from build123d import *

# Parameters (mm, degrees)
PAD008_DEPTH    = 21
POCKET020_DEPTH = 74.801
POCKET021_DEPTH = 1
CHAMFER008_SIZE = 0.99
POCKET022_DEPTH = 1
CHAMFER009_SIZE = 0.99
POCKET023_DEPTH = 74.801
CHAMFER010_SIZE = 4
FILLET003_R     = 6
FILLET004_R     = 5
SKETCH033_W     = 74.8
SKETCH033_H     = 11
PAD009_DEPTH    = 24
SKETCH034_R     = 3.15
POCKET024_DEPTH = 22.001
SKETCH035_R     = 7.5
POCKET025_DEPTH = 6
CHAMFER011_SIZE = 9
FILLET005_R     = 3
CHAMFER012_SIZE = 0.4


with BuildPart() as part:
    # Sketch028 → Pad008 (new body)
    with BuildSketch(Plane.XY):
        Polygon((-25.65, -11), (-25.65, 0.15), (35.45, 0.15), (35.45, -11), (42.3, -11), (42.3, 11), (-32.5, 11), (-32.5, -11), align=None)
    extrude(amount=PAD008_DEPTH)

    # Sketch029 (on Face7 of Pad008) → Pocket020 (cut, through all)
    with BuildSketch(Plane(origin=(-32.5, 0, 0), x_dir=(0, -1, 0), z_dir=(-1, 0, 0))):
        with BuildLine():
            ThreePointArc((3.35, 6.5), (5, 4.85), (6.65, 6.5))
            Line((6.65, 6.5), (6.65, 11.5))
            ThreePointArc((6.65, 11.5), (5, 13.15), (3.35, 11.5))
            Line((3.35, 6.5), (3.35, 11.5))
        make_face()
    extrude(amount=-POCKET020_DEPTH, mode=Mode.SUBTRACT)

    # Sketch030 (on Face10 of Pocket020) → Pocket021 (cut)
    with BuildSketch(Plane(origin=(-32.5, 0, 0), x_dir=(0, -1, 0), z_dir=(-1, 0, 0))):
        with BuildLine():
            ThreePointArc((8.65, 11.5), (5, 15.15), (1.35, 11.5))
            Line((1.35, 11.5), (1.35, 6.5))
            ThreePointArc((1.35, 6.5), (5, 2.85), (8.65, 6.5))
            Line((8.65, 11.5), (8.65, 6.5))
        make_face()
    extrude(amount=-POCKET021_DEPTH, mode=Mode.SUBTRACT)

    # Chamfer008
    chamfer008_edges = [part.edges().sort_by_distance(p)[0] for p in [
        (-32.5, -1.35, 9),
    ]]
    chamfer(chamfer008_edges, length=CHAMFER008_SIZE)

    # Sketch031 (on Face14 of Chamfer008) → Pocket022 (cut)
    with BuildSketch(Plane.YZ.offset(42.3)):
        with BuildLine():
            ThreePointArc((-1.35, 11.5), (-5, 15.15), (-8.65, 11.5))
            Line((-8.65, 11.5), (-8.65, 6.5))
            ThreePointArc((-8.65, 6.5), (-5, 2.85), (-1.35, 6.5))
            Line((-1.35, 11.5), (-1.35, 6.5))
        make_face()
    extrude(amount=-POCKET022_DEPTH, mode=Mode.SUBTRACT)

    # Chamfer009
    chamfer009_edges = [part.edges().sort_by_distance(p)[0] for p in [
        (42.3, -8.65, 9),
    ]]
    chamfer(chamfer009_edges, length=CHAMFER009_SIZE)

    # Sketch032 (on Face1 of Chamfer009) → Pocket023 (cut, through all)
    with BuildSketch(Plane.YZ.offset(42.3)):
        Polygon((0, 21), (-11, 21), (-11, 17), align=None)
    extrude(amount=-POCKET023_DEPTH, mode=Mode.SUBTRACT)

    # Chamfer010
    chamfer010_edges = [part.edges().sort_by_distance(p)[0] for p in [
        (38.875, -11, 0),
        (-29.075, -11, 0),
    ]]
    chamfer(chamfer010_edges, length=CHAMFER010_SIZE)

    # Fillet003
    fillet003_edges = [part.edges().sort_by_distance(p)[0] for p in [
        (-29.075, -11, 17),
        (38.875, -11, 17),
    ]]
    fillet(fillet003_edges, radius=FILLET003_R)

    # Fillet004
    fillet004_edges = [part.edges().sort_by_distance(p)[0] for p in [
        (-29.075, -11, 4),
        (-29.075, -7, 0),
        (38.875, -11, 4),
        (38.875, -7, 0),
    ]]
    fillet(fillet004_edges, radius=FILLET004_R)

    # Sketch033 (on Face8 of Fillet004) → Pad009 (join)
    with BuildSketch(Plane.XY.offset(21)):
        with Locations((4.9, 5.5)):
            Rectangle(SKETCH033_W, SKETCH033_H)
    extrude(amount=PAD009_DEPTH)

    # Sketch034 (on Face17 of Pad009) → Pocket024 (cut, through all)
    with BuildSketch(Plane(origin=(0, 11, 0), x_dir=(-1, 0, 0), z_dir=(0, 1, 0))):
        with Locations((-27.3, 33)):
            Circle(SKETCH034_R)
        with Locations((17.5, 33)):
            Circle(SKETCH034_R)
    extrude(amount=-POCKET024_DEPTH, mode=Mode.SUBTRACT)

    # Sketch035 (on Face16 of Pocket024) → Pocket025 (cut)
    with BuildSketch(Plane.XZ):
        with Locations((-17.5, 33)):
            Circle(SKETCH035_R)
        with Locations((27.3, 33)):
            Circle(SKETCH035_R)
    extrude(amount=-POCKET025_DEPTH, mode=Mode.SUBTRACT)

    # Chamfer011
    chamfer011_edges = [part.edges().sort_by_distance(p)[0] for p in [
        (-32.5, 5.5, 45),
        (42.3, 5.5, 45),
    ]]
    chamfer(chamfer011_edges, length=CHAMFER011_SIZE)

    # Fillet005
    fillet005_edges = [part.edges().sort_by_distance(p)[0] for p in [
        (-32.5, 5.5, 36),
        (-23.5, 5.5, 45),
        (33.3, 5.5, 45),
        (42.3, 5.5, 36),
    ]]
    fillet(fillet005_edges, radius=FILLET005_R)

    # Chamfer012
    chamfer012_edges = [part.edges().sort_by_distance(p)[0] for p in [
        (-32.271639, 11, 35.90541),
        (-28, 11, 40.5),
        (-23.40541, 11, 44.771639),
        (4.9, 11, 45),
        (33.20541, 11, 44.771639),
        (37.8, 11, 40.5),
        (42.071639, 11, 35.90541),
        (42.3, 11, 17.37868),
        (4.9, 11, 0),
        (-32.5, 11, 17.37868),
        (-14.35, 11, 33),
        (30.45, 11, 33),
        (-32.5, 3.035534, 0),
        (-25, 0, 33),
        (-14.35, 6, 33),
        (19.8, 0, 33),
        (30.45, 6, 33),
        (42.3, 3.035534, 0),
        (-25.65, -3.35, 9),
        (35.45, -3.35, 9),
        (-31.5, -3.35, 9),
        (41.3, -3.35, 9),
    ]]
    chamfer(chamfer012_edges, length=CHAMFER012_SIZE)


with BuildPart() as part_1:
    # Body004005 placement: moved
    add(part.part.moved(Location((0, 12, -20.5))))


solid = part_1.part
Could you check a few things on this model? Use its own coordinates, in mm. A direction names the side the tool comes from. Coordinates: 2 decimals unless noted, no trailing zeros. Write each loop counter-clockwise with the first axis right and the second up, starting at its lowest first coordinate (ties: lowest second). Pieces come first, ordered by that corner, then holes. Notation, with made-up numbers: (6, 23) - (16, 23) arc R15 ccw to (16, 38) - close; hole circle Ø2 at (44, -34). An arc over 180 degrees is marked (long way). Write item = value, one per line.
1) Suppose I cut it at C-C on z = 12.5. State how many separate pieces and enclosed holes the cut face has, plus the area to 3 significant figures.
Result set:
separate_pieces = 3
enclosed_holes = 0
area = 579 mm2
2) For faces 4 (the flat face through (-31.5, 4.6, -11.4)), 5 (the cylindrical face through (38.34, 7.04, -15.65)), 6 (the flat face through (4, 12.15, -10)), which set-ups out of +Z, -Z, +X, -X, +Y, -Y let a thin tool reach every point of the face, with its end or its side?
Result set:
face_4 = -X
face_5 = +X, -X
face_6 = -Z, -Y
3) We'd pull the mould along Y, two halves only. Please class faces 1 (the flat face through (4, 17, -20.5)), 2 (the flat face through (-32.3, 3.15, -18.37)), 3 (the conical face through (41.01, 7.04, -7.24)): +Y half, -Y half, draft (parallel to the pull), parting line (faces both ways), or undercut.
Result set:
face_1 = draft
face_2 = -Y half
face_3 = undercut
4) Suppose I cut it at A-A on x = -17.5. Please give me the cut outline in (y, z), plus the area to 3 significant figures.
Result set:
outline = (12, 0.5) - (12.15, 0.5) - (12.15, -20.5) - (22.6, -20.5) - (23, -20.1) - (23, 8.95) - (22.6, 9.35) - (18.4, 9.35) - (18, 8.95) - (18, 5) - (12.4, 5) - (12, 4.6) - close; (12, 20.4) - (12.4, 20) - (18, 20) - (18, 16.05) - (18.4, 15.65) - (22.6, 15.65) - (23, 16.05) - (23, 24.1) - (22.6, 24.5) - (12, 24.5) - close
area = 370 mm2
5) Suppose I cut it at D-D on x = -28. Please give me the cut outline in (y, z).
Result set:
outline = (1, -14.43) arc R5 ccw to (2.46, -17.96) - (3.54, -19.04) arc R5 ccw to (7.07, -20.5) - (22.6, -20.5) - (23, -20.1) - (23, 19.43) - (22.6, 20) - (12, 20) - (12, 0.5) - (4.95, -2.06) arc R6 ccw to (1, -7.7) - close; hole (5.35, -14) arc R1.65 ccw to (8.65, -14) - (8.65, -9) arc R1.65 ccw to (5.35, -9) - close
6) Please list where these lines run through material, in increasing order: line 1 (Z direction, x = 27.3, y = 21.45); line 2 (X direction, y = 3.5, z = -11); line 3 (X direction, y = 11.75, z = -11.5). Write a range as [from, to].
Result set:
line_1 = [-20.5, 9.35], [15.65, 24.5]
line_2 = [-31.5, -25.65], [35.45, 41.3]
line_3 = [-32.5, -25.65], [35.45, 42.3]
7) Suppose I cut it at B-B on y = 15. Please give me the cut outline in (x, z).
Result set:
outline = (-32.5, -20.1) - (-32.1, -20.5) - (41.9, -20.5) - (42.3, -20.1) - (42.3, 14.26) arc R3 ccw to (41.42, 16.38) - (34.18, 23.62) arc R3 ccw to (32.06, 24.5) - (-22.26, 24.5) arc R3 ccw to (-24.38, 23.62) - (-31.62, 16.38) arc R3 ccw to (-32.5, 14.26) - close; hole circle Ø15 at (-17.5, 12.5); hole circle Ø15 at (27.3, 12.5)
8) Will these pins go through, and if not, where does the flat tip stop? pin 1 Ø12 at (x, z) = (17.5, 12) entering from -Y; pin 2 Ø23 at (x, z) = (-8.5, -14.5) entering from -Y; pin 3 Ø10 at (y, z) = (6.5, 5) entering from -X; pin 4 Ø7 at (x, z) = (-17.5, 12.5) entering from -Y.
Result set:
pin_1 = 12
pin_2 = 12.15
pin_3 = through
pin_4 = 18.05
